Could you check a few things on this model? Use its own coordinates, in mm. Coordinates: 2 decimals unless noted, no trailing zeros. Loops run counter-clockwise (first coordinate to the right, second up) from the corner with the lowest first, then second, coordinate; pieces in that order, holes last. Notation, with made-up numbers: (7, -5.5) - (64, -5.5) arc R28 cw to (64, 15.5) - close; hole circle Ø4 at (6, 40). An arc over 180 degrees is marked (long way). Use CSV: the item, a comma, the result in double quotes.
from build123d import *

# Parameters (mm, degrees)
BOSS_EXTRUDE1_DEPTH = 32.65
SKETCH2_R           = 9.8
SKETCH2_R_2         = 9.3
BOSS_EXTRUDE2_DEPTH = 5
LPATTERN1_COUNT     = 2
LPATTERN1_PITCH     = 40


with BuildPart() as part:
    # Sketch1 → Boss-Extrude1 (new body, symmetric)
    with BuildSketch(Plane.XY):
        with BuildLine():
            Line((-0.361769768, 9.693251396), (-0.361769768, 9.292960919))
            ThreePointArc((-0.361769768, 9.292960919), (-9.292960919, -0.361769768), (0.361769768, -9.292960919))
            Line((0.361769768, -9.292960919), (0.361769768, -9.693251396))
            ThreePointArc((0.361769768, -9.693251396), (-9.693251396, -0.361769768), (-0.361769768, 9.693251396))
        make_face()
    extrude(amount=BOSS_EXTRUDE1_DEPTH, both=True)

    # Sketch2 → Boss-Extrude2 (add, symmetric)
    with BuildSketch(Plane.XY.offset(20)):
        Circle(SKETCH2_R)
        Circle(SKETCH2_R_2, mode=Mode.SUBTRACT)
    boss_extrude2 = extrude(amount=BOSS_EXTRUDE2_DEPTH, both=True)

    # LPattern1: Boss-Extrude2 ×2
    with Locations(*[(0, 0, -i * LPATTERN1_PITCH) for i in range(1, LPATTERN1_COUNT)]):
        add(boss_extrude2)


solid = part.part
(1) Suppose I cut it at B-B (x = -7.25). Write out the boundary of the cut face in (y, z).
Computed:
outline,"(-6.59, -25) - (-6.44, -25) - (-6.44, -32.65) - (-5.82, -32.65) - (-5.82, 32.65) - (-6.44, 32.65) - (-6.44, 25) - (-6.59, 25) - (-6.59, 15) - (-6.44, 15) - (-6.44, -15) - (-6.59, -15) - close; (5.82, -32.65) - (6.44, -32.65) - (6.44, -25) - (6.59, -25) - (6.59, -15) - (6.44, -15) - (6.44, 15) - (6.59, 15) - (6.59, 25) - (6.44, 25) - (6.44, 32.65) - (5.82, 32.65) - close"
(2) Suppose I cut it at D-D (y = 8.25). Write out the boundary of the cut face in (x, z), plus the area to 3 significant figures.
Computed:
outline,"(-5.29, -25) - (-5.1, -25) - (-5.1, -32.65) - (-4.29, -32.65) - (-4.29, 32.65) - (-5.1, 32.65) - (-5.1, 25) - (-5.29, 25) - (-5.29, 15) - (-5.1, 15) - (-5.1, -15) - (-5.29, -15) - close; (4.29, -25) - (5.29, -25) - (5.29, -15) - (4.29, -15) - close; (4.29, 15) - (5.29, 15) - (5.29, 25) - (4.29, 25) - close"
area,"76.5 mm²"
(3) Suppose I cut it at C-C (x = 5.5). Write out the boundary of the cut face in (y, z).
Computed:
outline,"(-8.11, -25) - (-7.5, -25) - (-7.5, -15) - (-8.11, -15) - close; (-8.11, 15) - (-7.5, 15) - (-7.5, 25) - (-8.11, 25) - close; (7.5, -25) - (8.11, -25) - (8.11, -15) - (7.5, -15) - close; (7.5, 15) - (8.11, 15) - (8.11, 25) - (7.5, 25) - close"
(4) Please list where these lines run through material, in increasing order: line 1 (X direction, y = -0.5, z = 21); line 2 (Y direction, x = 0, z = 1).
Computed:
line 1,"x = -9.79 to -9.29, 9.29 to 9.79"
line 2,"y = -9.7 to -9.3"
(5) Thinking about a two-plate mould opening in Z: for faces 1 (the face through (-2.124, -9.567, -19.93)), 2 (the face through (-9.5, 0, 32.65)), 3 (the face through (-9.683, -0.575, 0.21)), which applies, +Z half, -Z half, draft (parallel to the pull), parting line (faces both ways), or undercut?
Computed:
face 1,"draft"
face 2,"+Z half"
face 3,"undercut"
(6) Will these pins go through, and if not, where does the flat tip stop? pin 1 (3 mm diameter, centred on y = 4.5, z = -25.5, fed in from -X); pin 2 (1 mm diameter, centred on y = -4, z = 22.5, fed in from +X); pin 3 (8 mm diameter, centred on y = 8, z = 25, fed in from -X).
Computed:
pin 1,"stops at x = -9.3"
pin 2,"stops at x = 9.15"
pin 3,"stops at x = -8.95"
(7) Suppose I cut it at A-A (y = 0). Write out the boundary of the cut face in (x, z), plus the area to 3 significant figures.
Computed:
outline,"(-9.8, -25) - (-9.7, -25) - (-9.7, -32.65) - (-9.3, -32.65) - (-9.3, 32.65) - (-9.7, 32.65) - (-9.7, 25) - (-9.8, 25) - (-9.8, 15) - (-9.7, 15) - (-9.7, -15) - (-9.8, -15) - close; (9.3, -25) - (9.8, -25) - (9.8, -15) - (9.3, -15) - close; (9.3, 15) - (9.8, 15) - (9.8, 25) - (9.3, 25) - close"
area,"38.1 mm²"
